The model under review builds one solid part; all positions refer to its coordinate system, in mm. A direction names the side the tool comes from. Coordinates: 2 decimals unless noted, no trailing zeros. Loops run counter-clockwise (first coordinate to the right, second up) from the corner with the lowest first, then second, coordinate; pieces in that order, holes last. Notation, with made-up numbers: (55.5, 78) - (97.5, 78) arc R16 ccw to (97.5, 107) - close; hole circle Ø1 at (-28.5, 56.25). An arc over 180 degrees is marked (long way). One line per item, written item: value. Start each with the question number.
1. We need section B-B, the plane z = 9.5. Give the boundary of the cut face in (x, y).
2. Mouldability with a two-part tool opening along Y and no side actions: class faces 1 (the face through (0, -2, 44)), 2 (the face through (1, 0, 42.5)), 3 (the face through (0.03, 0.05, -48.75)) as +Y half, -Y half, draft (parallel to the pull), parting line (faces both ways), or undercut.
3. To check wall thickness, follow line 1 (Z direction, x = -0.1, y = 0); line 2 (Z direction, x = 0.25, y = -0.75); line 3 (Z direction, x = -0.05, y = 1.1). State the ranges of each line that lie inside material, in increasing order.
4. For faces 4 (the face through (0.03, 0.845, 48.421)), 5 (the face through (1, 0, -42.5)), list the 3-axis set-ups (+Z, -Z, +X, -X, +Y, -Y) from which the entire face can be reached by the end or side of a thin tool; tool diameter is ignored.
5. Insertion check: P1, Ø1.5, axis at x = 1, y = 1.5, coming from the +Z side; P2, Ø1.5, axis at x = 1.5, z = 32, coming from the -Y side; P3, Ø1.5, axis at y = 0.5, z = 29.5, coming from the -X side; P4, Ø1.5, axis at x = -0.5, z = 39, coming from the +Y side. Each pin has a flat end and moves straight along its axis. Give the tip position at first contact, or say it passes through.
6. We need section A-A, the plane z = 47.5. Give the boundary of the cut face in (x, y).
from build123d import *

# Parameters (mm, degrees)
SKETCH1_R           = 0.6
BOSS_EXTRUDE1_DEPTH = 42.5
SKETCH2_R           = 2
BOSS_EXTRUDE2_DEPTH = 5
SKETCH6_R           = 1.25
CUT_EXTRUDE2_DEPTH  = 51.124844139


with BuildPart() as part:
    # Sketch1 → Boss-Extrude1 (new, symmetric)
    with BuildSketch(Plane.XY):
        Circle(SKETCH1_R)
    extrude(amount=BOSS_EXTRUDE1_DEPTH, both=True)

    # Sketch2 → Boss-Extrude2 (add)
    with BuildSketch(Plane.XY.offset(42.5)):
        Circle(SKETCH2_R)
    boss_extrude2 = extrude(amount=BOSS_EXTRUDE2_DEPTH)

    # Sketch3 → Revolve1 (revolve)
    with BuildSketch(Plane(origin=(0, 0, 0), x_dir=(1, 0, 0), z_dir=(0, 1, 0))):
        with BuildLine():
            Line((0, -45), (0, -50))
            ThreePointArc((0, -50), (2.5, -47.5), (0, -45))
        make_face()
    revolve1 = revolve(axis=Axis((0, 0, 45), (0, 0, 1)))

    # Sketch6 → Cut-Extrude2 (cut, symmetric)
    with BuildSketch(Plane(origin=(0, 0, 0), x_dir=(0, 0, -1), z_dir=(1, 0, 0))):
        with Locations((-47.5, 0)):
            Circle(SKETCH6_R)
    cut_extrude2 = extrude(amount=CUT_EXTRUDE2_DEPTH, both=True, mode=Mode.SUBTRACT)

    # Mirror1: Boss-Extrude2, Revolve1, Cut-Extrude2 across plane
    add(boss_extrude2.mirror(Plane.XY))
    add(revolve1.mirror(Plane.XY))
    add(cut_extrude2.mirror(Plane.XY), mode=Mode.SUBTRACT)


solid = part.part
Findings below:
1. outline: circle Ø1.2 at (0, 0)
2. face 1: parting line
2. face 2: draft
2. face 3: undercut
3. line 1: -50 to -48.75, -46.25 to 46.25, 48.75 to 50
3. line 2: -49.87 to -48.5, -46.5 to -42.5, 42.5 to 46.5, 48.5 to 49.87
3. line 3: -49.74 to -48.09, -46.91 to -42.5, 42.5 to 46.91, 48.09 to 49.74
4. face 4: +X, -X
4. face 5: none
5. P1: z = 49.77
5. P2: through
5. P3: x = -0.6
5. P4: y = 0.6
6. outline: (-2.17, -1.25) arc R2.5 ccw to (2.17, -1.25) - close; (-2.17, 1.25) - (2.17, 1.25) arc R2.5 ccw to start
